Verification items for the finished model (mm, model axes). Face numbers are marked on the shaded views. Give positions to 0.01 mm unless a question says otherwise; leave off trailing zeros. Write each loop counter-clockwise with the first axis right and the second up, starting at its lowest first coordinate (ties: lowest second). Pieces come first, ordered by that corner, then holes. Notation, with made-up numbers: M 17.25,13 L 26.25,13 A18 ccw 26.25,33 Z; hole C 75.5,72 d3. An arc over 180 degrees is marked long. Answer as a JSON object with one key per item and string values.
Autodesk Inventor part; units mm, degrees
ref_plane "YZ Plane" through (0, 0, 0) normal (1, 0, 0) x (0, 1, 0)
ref_plane "XZ Plane" through (0, 0, 0) normal (0, 1, 0) x (-1, 0, 0)
ref_plane "XY Plane" through (0, 0, 0) normal (0, 0, 1) x (1, 0, 0)
sketch "Sketch1" plane through (0, 0, 0) normal (0, 0, 1) x (1, 0, 0)
  line L0 (0, 0) -> (58.8772, 0)
  line L1 (58.8772, 0) -> (58.8772, 129.921)
  line L2 (58.8772, 129.921) -> (0, 129.921)
  line L3 (0, 129.921) -> (0, 0)
  dimension "d0" = 58.8772
  dimension "d1" = 129.921
extrude "Stock Bar" add sketch "Sketch1" along normal blind 6.35
fillet "Round Edges" radius 3.6068 2 edges at (0, 129.921, 3.175) (58.8772, 129.921, 3.175)
sketch "Sketch2" plane through (0, 0, 6.35) normal (0, 0, 1) x (1, 0, 0)
  circle A0 centre (29.4386, 99.441) radius 19.304
  line L0 (58.8772, 129.921) -> (0, 129.921)
  line L1 (0, 129.921) -> (0, 0)
  line L2 (58.8772, 0) -> (58.8772, 129.921)
  line L3 (29.4386, 129.921) -> (29.4386, 0)
  line L4 (0, 0) -> (58.8772, 0)
  dimension "d4" = 38.608
  dimension "d32" = 99.441
extrude "Motor Hole" cut sketch "Sketch2" against normal blind 6.35 contours A0 L3 | L3 A0
sketch "Sketch3" plane through (0, 0, 6.35) normal (0, 0, 1) x (1, 0, 0)
  circle A0 centre (5.8166, 123.0122) radius 2.6035
  line L0 (58.8772, 129.921) -> (0, 129.921)
  line L1 (0, 129.921) -> (0, 0)
  circle A1 centre (5.8166, 75.8698) radius 2.6035
  circle A2 centre (52.959, 123.0122) radius 2.6035
  circle A3 centre (52.959, 75.8698) radius 2.6035
  line L2 (0, 0) -> (58.8772, 0)
  dimension "d10" = 5.207
  dimension "d15" = 47.1424
  dimension "d18" = 47.1424
  dimension "d33" = 123.0122
  dimension "d34" = 5.8166
extrude "Motor Mounting Holes" cut sketch "Sketch3" against normal blind 6.35
sketch "Sketch4" plane through (0, 0, 6.35) normal (0, 0, 1) x (1, 0, 0)
  circle A0 centre (15.875, 9.525) radius 3.302
  circle A1 centre (43.0022, 9.525) radius 3.302
  line L0 (0, 0) -> (58.8772, 0)
  line L1 (58.8772, 0) -> (58.8772, 126.3142)
  line L2 (0, 126.3142) -> (0, 0)
  dimension "d24" = 6.604
  dimension "d25" = 6.604
  dimension "d26" = 9.525
  dimension "d27" = 9.525
  dimension "d28" = 15.875
  dimension "d29" = 15.875
extrude "Motor Support Mounting Holes" cut sketch "Sketch4" against normal blind 25.4
properties part number "Motor Support" material "Aluminum 6061"
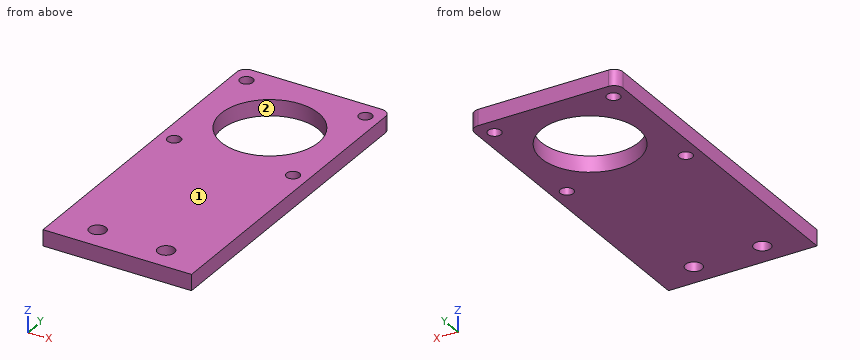
1) Section check C-C on z = 4.5. Record the boundary of the cut face in (x, y) (1 decimal).
Completed:
{"outline": "M 0,0 L 58.9,0 L 58.9,126.3 A3.6 ccw 55.3,129.9 L 3.6,129.9 A3.6 ccw 0,126.3 Z; hole C 5.8,75.9 d5.2; hole C 5.8,123 d5.2; hole C 29.4,99.4 d38.6; hole C 15.9,9.5 d6.6; hole C 43,9.5 d6.6; hole C 53,75.9 d5.2; hole C 53,123 d5.2"}
2) Section check A-A on x = 29. Record the boundary of the cut face in (y, z).
Completed:
{"outline": "M 0,0 L 80.14,0 L 80.14,6.35 L 0,6.35 Z; M 118.74,0 L 129.92,0 L 129.92,6.35 L 118.74,6.35 Z"}
3) Release check for a two-part mould opening along Y. For the marked faces 1 and 2 record: pulls with the +Y half, pulls with the -Y half, needs draft (parallel to the pull), parting line crosses it, or undercut.
Completed:
{"face 1": "needs draft", "face 2": "undercut"}
4) Section check D-D on x = 7. Record the boundary of the cut face in (y, z).
Completed:
{"outline": "M 0,0 L 73.55,0 L 73.55,6.35 L 0,6.35 Z; M 78.19,0 L 120.69,0 L 120.69,6.35 L 78.19,6.35 Z; M 125.33,0 L 129.92,0 L 129.92,6.35 L 125.33,6.35 Z"}
5) Section check B-B on y = 11. Record the boundary of the cut face in (x, z).
Completed:
{"outline": "M 0,0 L 12.92,0 L 12.92,6.35 L 0,6.35 Z; M 18.83,0 L 40.05,0 L 40.05,6.35 L 18.83,6.35 Z; M 45.96,0 L 58.88,0 L 58.88,6.35 L 45.96,6.35 Z"}
6) Go/stop test with a flat-tipped pin: pin 1 (4 mm diameter, centred on x = 5.82, y = 75.87, fed in from -Z). Record where the tip stops, or that it passes through.
Completed:
{"pin 1": "passes through"}
7) Thickness scan on L1, parallel to X at y = 100, z = 4; L2, parallel to Y at x = 4, z = 2.75; L3, parallel to Y at x = 6.5, z = 5.5. Record the ranges inside material, lowest first.
Completed:
{"L1": "x = 0 to 10.14, 48.73 to 58.88", "L2": "y = 0 to 74, 77.73 to 121.15, 124.88 to 129.92", "L3": "y = 0 to 73.36, 78.38 to 120.5, 125.52 to 129.92"}
